The listing builds one solid part. Answer for the finished solid, in the listing's coordinates (mm). A direction names the side the tool comes from. Round coordinates to 2 decimals unless told otherwise and drop trailing zeros. Order: outer loops, then holes, each group sorted by start corner. A loop starts at its lowest first (then second) coordinate and runs counter-clockwise, first axis right, second up. Notation, with made-up numbers: M 42.5,-16.5 L 58.5,-16.5 A31 cw 58.5,7.5 Z; hole C 15.5,87 d1. An arc over 180 degrees is marked long. Put each result on its own line as item: value. Start each with the question number.
1. Consider line 1 (X direction, y = 9.25, z = 83.15); line 2 (Z direction, x = 105.5, y = 1.6); line 3 (Z direction, x = 138.5, y = 7.25). Determine where each line is inside the solid, lowest interval first.
2. Each of these flat-tipped pins is pushed along its axis until it touches: pin 1 Ø6 at (x, z) = (188.5, 112) entering from -Y; pin 2 Ø4 at (x, z) = (20.5, 70.5) entering from -Y; pin 3 Ø1.5 at (y, z) = (3, 25) entering from -X; pin 4 Ø1.9 at (x, z) = (20.5, 10.5) entering from -Y. Where does it stop, or does it pass through?
3. The part is cut by section D-D (x = 5). Give the vertices of the cut face in (y, z), then the cut area to 3 significant figures.
4. The part is cut by section A-A (x = 34.5). Give the vertices of the cut face in (y, z).
5. The part is cut by section B-B (z = 83.15). Give the vertices of the cut face in (x, y), then the cut area to 3 significant figures.
6. Which of the six approach directions +Z, -Z, +X, -X, +Y, -Y give full straight-line access (tool end or side, diameter ignored) to faces 1 (the face through (147, 5, 75.5)), 2 (the face through (179.1, 10, 74)), 3 (the face through (185, 12.5, 74)), 4 (the face through (53, 4, 91))?
7. The part is cut by section C-C (z = 131). Give the vertices of the cut face in (x, y).
8. The mould has two halves that part along X. Classify faces 5 (the face through (0, 9, 74)), 6 (the face through (97, 5, 150)), 7 (the face through (65, 5, 86)): +X half, -X half, draft (parallel to the pull), parting line (faces both ways), or undercut.
from build123d import *

# Parameters (mm, degrees)
PLATEFRAME_DEPTH          = 150
SKETCH3_R                 = 2.15
HOLESUPPORT_DEPTH         = 7.5
SKETCH4_R                 = 4.15
SKETCH4_R_2               = 2.15
CYLINDRICALSUPPORTS_DEPTH = 12.5
SKETCH5_W                 = 101
SKETCH5_H                 = 81
SKETCH5_W_2               = 58
SKETCH5_H_2               = 73
SKETCH5_W_3               = 73
SKETCH5_H_3               = 58
ITEMLAYOUT_DEPTH          = 5
SKETCH6_R                 = 1.6
JETSONBASEHOLES_DEPTH     = 2.5
SKETCH7_W                 = 76.1
SKETCH7_H                 = 56.5
OPENHOLE_DEPTH            = 8.5


with BuildPart() as part:
    # Sketch2 → PlateFrame (new body)
    with BuildSketch(Plane.XY):
        Polygon((179.1, 12.5), (191.6, 12.5), (191.6, 5), (184.1, 5), (184.1, 0), (7.5, 0), (7.5, 5), (0, 5), (0, 12.5), (12.5, 12.5), (12.5, 7.5), (179.1, 7.5), align=None)
    extrude(amount=PLATEFRAME_DEPTH)

    # Sketch3 → HoleSupport (cut)
    with BuildSketch(Plane(origin=(0, 12.5, 0), x_dir=(1, 0, 0), z_dir=(0, 1, 0))):
        with Locations((5, -66.85)):
            Circle(SKETCH3_R)
        with Locations((5, -83.15)):
            Circle(SKETCH3_R)
        with Locations((186.6, -66.85)):
            Circle(SKETCH3_R)
        with Locations((186.6, -83.15)):
            Circle(SKETCH3_R)
    extrude(amount=-HOLESUPPORT_DEPTH, mode=Mode.SUBTRACT)

    # Sketch4 → CylindricalSupports (add)
    with BuildSketch(Plane(origin=(0, 12.5, 0), x_dir=(1, 0, 0), z_dir=(0, 1, 0))):
        with Locations((186.6, -66.85)):
            Circle(SKETCH4_R)
        with Locations((186.6, -66.85)):
            Circle(SKETCH4_R_2, mode=Mode.SUBTRACT)
        with Locations((186.6, -83.15)):
            Circle(SKETCH4_R)
        with Locations((186.6, -83.15)):
            Circle(SKETCH4_R_2, mode=Mode.SUBTRACT)
        with Locations((5, -66.85)):
            Circle(SKETCH4_R)
        with Locations((5, -66.85)):
            Circle(SKETCH4_R_2, mode=Mode.SUBTRACT)
        with Locations((5, -83.15)):
            Circle(SKETCH4_R)
        with Locations((5, -83.15)):
            Circle(SKETCH4_R_2, mode=Mode.SUBTRACT)
    extrude(amount=-CYLINDRICALSUPPORTS_DEPTH)

    # Sketch5 → ItemLayout (cut)
    with BuildSketch(Plane(origin=(0, 7.5, 0), x_dir=(1, 0, 0), z_dir=(0, 1, 0))):
        with Locations((65.5, -45.5)):
            Rectangle(SKETCH5_W, SKETCH5_H)
        with Locations((147.6, -39)):
            Rectangle(SKETCH5_W_2, SKETCH5_H_2)
        with Locations((132.6, -118.5)):
            Rectangle(SKETCH5_W_3, SKETCH5_H_3)
    extrude(amount=-ITEMLAYOUT_DEPTH, mode=Mode.SUBTRACT)

    # Sketch6 → JetsonBaseHoles (cut)
    with BuildSketch(Plane(origin=(0, 2.5, 0), x_dir=(1, 0, 0), z_dir=(0, 1, 0))):
        with Locations((20.5, -10.5)):
            Circle(SKETCH6_R)
        with Locations((20.5, -70.5)):
            Circle(SKETCH6_R)
        with Locations((105.5, -70.5)):
            Circle(SKETCH6_R)
        with Locations((105.5, -10.5)):
            Circle(SKETCH6_R)
    extrude(amount=-JETSONBASEHOLES_DEPTH, mode=Mode.SUBTRACT)

    # Sketch7 → OpenHole (cut, through all)
    with BuildSketch(Plane(origin=(0, 7.5, 0), x_dir=(1, 0, 0), z_dir=(0, 1, 0))):
        with Locations((53.05, -119.25)):
            Rectangle(SKETCH7_W, SKETCH7_H)
    extrude(amount=-OPENHOLE_DEPTH, mode=Mode.SUBTRACT)


solid = part.part
Resolved:
1. line 1: 0 to 2.85, 7.15 to 12.5, 179.1 to 184.45, 188.75 to 191.6
1. line 2: 0 to 8.9, 12.1 to 68.9, 72.1 to 150
1. line 3: 0 to 2.5, 75.5 to 89.5, 147.5 to 150
2. pin 1: y = 5
2. pin 2: y = 0
2. pin 3: x = 7.5
2. pin 4: through
3. outline: M 0,62.7 L 5,62.7 L 5,0 L 12.5,0 L 12.5,64.7 L 0,64.7 Z; M 0,69 L 12.5,69 L 12.5,81 L 0,81 L 0,79 L 5,79 L 5,71 L 0,71 Z; M 0,85.3 L 12.5,85.3 L 12.5,150 L 5,150 L 5,87.3 L 0,87.3 Z
3. area: 1,100 mm2
4. outline: M 0,0 L 7.5,0 L 7.5,5 L 2.5,5 L 2.5,86 L 7.5,86 L 7.5,91 L 0,91 Z; M 0,147.5 L 7.5,147.5 L 7.5,150 L 0,150 Z
5. outline: M 0,5 L 0.85,5 L 0.85,0 L 2.85,0 L 2.85,12.5 L 0,12.5 Z; M 7.15,0 L 184.45,0 L 184.45,12.5 L 179.1,12.5 L 179.1,7.5 L 116,7.5 L 116,2.5 L 15,2.5 L 15,7.5 L 12.5,7.5 L 12.5,12.5 L 7.15,12.5 Z; M 188.75,0 L 190.75,0 L 190.75,5 L 191.6,5 L 191.6,12.5 L 188.75,12.5 Z
5. area: 941 mm2
6. face 1: +Y
6. face 2: +Z, -Z, +Y
6. face 3: +Z, -Z, +X, -X, +Y
6. face 4: +Y, -Y
7. outline: M 0,5 L 7.5,5 L 7.5,0 L 15,0 L 15,7.5 L 12.5,7.5 L 12.5,12.5 L 0,12.5 Z; M 91.1,0 L 184.1,0 L 184.1,5 L 191.6,5 L 191.6,12.5 L 179.1,12.5 L 179.1,7.5 L 169.1,7.5 L 169.1,2.5 L 96.1,2.5 L 96.1,7.5 L 91.1,7.5 Z
8. face 5: -X half
8. face 6: draft
8. face 7: undercut
